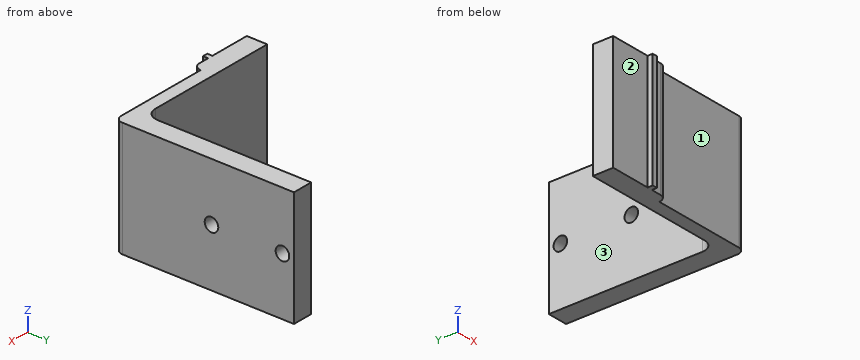
Autodesk Fusion 360 part; units mm, degrees
sketch "Sketch1" plane through (0, 0, 0) normal (0, 0, 1) x (1, 0, 0)
  line L0 (0, 0) -> (65, 0)
  line L1 (65, 0) -> (65, 8)
  line L2 (65, 8) -> (0, 8)
  line L3 (0, 8) -> (0, 0)
  line L4 (65, 0) -> (57, 0)
  line L5 (57, 0) -> (57, 73)
  line L6 (57, 73) -> (65, 73)
  line L7 (65, 73) -> (65, 0)
  line L8 (65, 0) -> (25, 0)
  line L9 (25, 0) -> (25, 3)
  line L10 (25, 3) -> (65, 3)
  line L11 (65, 3) -> (65, 0)
  dimension "d1" = 65
  dimension "d2" = 8
  dimension "d3" = 8
  dimension "d4" = 73
  dimension "d37" = 40
  dimension "d38" = 3
extrude "Extrude1" add sketch "Sketch1" along normal blind 45
sketch "Sketch2" plane through (0, 0, 0) normal (0, -1, 0) x (1, 0, 0)
  line L0 (0, 0) -> (65, 0)
  line L1 (65, 0) -> (65, 45)
  line L2 (65, 45) -> (0, 45)
  line L3 (0, 45) -> (0, 0)
  line L4 (16, 0) -> (18, 0)
  line L5 (18, 0) -> (18, 60)
  line L6 (18, 60) -> (16, 60)
  line L7 (16, 60) -> (16, 0)
  dimension "d7" = 2
  dimension "d8" = 60
  dimension "d9" = 16
extrude "Extrude2" add sketch "Sketch2" along normal blind 2 contours L0 L2 L4 L5 L7
sketch "Sketch3" plane through (57, 0, 0) normal (-1, 0, 0) x (0, -1, 0)
  line L0 (-73, 0) -> (-8, 0)
  line L1 (-8, 0) -> (-8, 45)
  line L2 (-8, 45) -> (-73, 45)
  line L3 (-73, 45) -> (-73, 0)
  line L4 (-73, 22.5) -> (-8.58, 22.5) construction
  circle A0 centre (-68.5, 22.5) radius 2
  circle A1 centre (-40.79, 22.5) radius 2
  circle A2 centre (-68.5, 22.5) radius 2.65
  circle A3 centre (-40.79, 22.5) radius 2.65
  line L5 (-73, 0) -> (-18, 0)
  line L6 (-18, 0) -> (-18, 10)
  line L7 (-18, 10) -> (-73, 10)
  line L8 (-73, 10) -> (-73, 0)
  dimension "d25" = 4
  dimension "d27" = 4
  dimension "d28" = 4.5
  dimension "d29" = 27.71
  dimension "d30" = 5.3
  dimension "d31" = 5.3
  dimension "d49" = 55
  dimension "d50" = 10
extrude "Extrude5" cut sketch "Sketch3" against normal blind 8 contours A0 | A1
extrude "Extrude6" cut sketch "Sketch3" against normal blind 8 contours A2 | A3
extrude "Extrude7" cut sketch "Sketch1" along normal blind 70 contours L0 L5 L8 L9 L10 | L0 L1 L4 L5 L7 L8 L10 L11
fillet "Fillet1" radius 3 1 edges at (25, 0, 22.5)
fillet "Fillet2" radius 3 1 edges at (65, 3, 22.5)
fillet "Fillet3" radius 5 1 edges at (57, 8, 22.5)
equation "d1 = 39 mm + 5 mm + 16 mm + 5 mm"
equation "d4 = 48 mm + 5 mm + 10 mm + 10 mm"
Check sheet for the modelled part. Datum: model origin and axes. Units: mm. Face numbers are marked on the shaded views. A direction names the side the tool comes from. Round coordinates to 2 decimals unless told otherwise and drop trailing zeros. Order: outer loops, then holes, each group sorted by start corner. A loop starts at its lowest first (then second) coordinate and runs counter-clockwise, first axis right, second up.
(1) Access from +Z, -Z, +X, -X, +Y, -Y to the whole of each face (thin tool, end or side, straight path). Record for the marked faces 1, 2 and 3.
(2) Cross-section at B-B, the plane y = 40.79. Enter the section's corners in (x, z).
(3) Cross-section at D-D, the plane x = 27. Enter the section's corners in (y, z), and give its area (3 significant figures).
(4) Go/stop test with flat-tipped pins: P1, Ø1, axis at y = 58.5, z = 28.5, coming from the -X side; P2, Ø1, axis at x = 46.5, z = 31, coming from the +Y side; P3, Ø1.2, axis at x = 20.5, z = 31.5, coming from the -Y side; P4, Ø3, axis at y = 68.5, z = 22.5, coming from the -X side. Record where each tip stops, or that it passes through.
(5) Cross-section at A-A, the plane z = 22.5. State how many separate pieces and enclosed holes the cut face has, and give its area (3 significant figures).
(6) Scan lines: probe 1 along Z at (x, y) = (58.75, 68.5); probe 2 along Y at (x, z) = (63, 22); probe 3 along X at (y, z) = (55, 10). Record each from-to range of solid material in increasing order.
Check sheet entries:
1. face 1: +Z, -Z, +X, -Y
1. face 2: +Z, -Z, -X, -Y
1. face 3: +Z, -Z, -X, +Y
2. outline: (57, 0) - (65, 0) - (65, 19.85) - (57, 19.85) - close; (57, 25.15) - (65, 25.15) - (65, 45) - (57, 45) - close
3. outline: (3, 0) - (8, 0) - (8, 45) - (3, 45) - close
3. area: 225 mm2
4. P1: stops at x = 57
4. P2: stops at y = 8
4. P3: stops at y = 0
4. P4: passes through
5. separate pieces: 3
5. enclosed holes: 0
5. area: 841 mm2
6. probe 1: z = 0 to 19.85, 25.15 to 45
6. probe 2: y = 3.17 to 38.19, 43.39 to 65.9, 71.1 to 73
6. probe 3: x = 57 to 65
